Can you work these out from the model? Positions are in its coordinate system, mm. Give positions to 0.01 mm unless a question says otherwise; leave off trailing zeros. Loops run counter-clockwise (first coordinate to the right, second up) from the corner with the lowest first, then second, coordinate; pieces in that order, holes last. Notation, with made-up numbers: (-36, 37.25) -> (-5, 37.25) arc R37 cw to (-5, 76.25) -> close; hole circle Ø5 at (32, -20). An arc over 180 degrees is marked (long way). One line per question, with ' | ' between items.
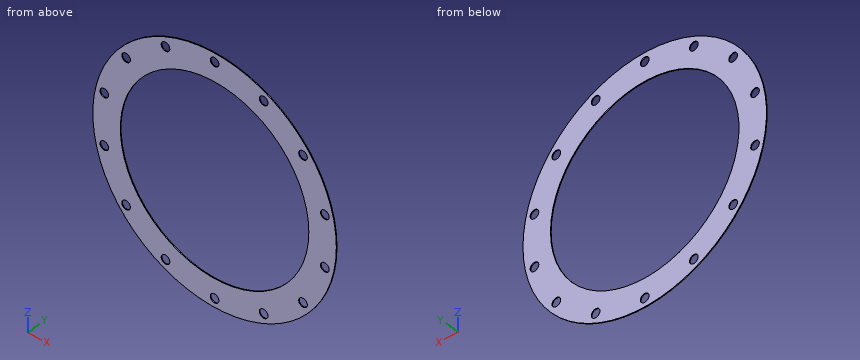
from build123d import *

# Parameters (mm, degrees)
F0_R     = 492.125
F0_R_2   = 17.4625
F0_R_3   = 381
F1_DEPTH = 3.175


with BuildPart() as f1:
    # F0 (on Front) → F1 (new body)
    with BuildSketch(Plane.XZ):
        Circle(F0_R)
        with Locations((-357.453354, -285.059537)):
            Circle(F0_R_2, mode=Mode.SUBTRACT)
        with Locations((-198.371646, -411.922966)):
            Circle(F0_R_2, mode=Mode.SUBTRACT)
        with Locations((0, -457.2)):
            Circle(F0_R_2, mode=Mode.SUBTRACT)
        with Locations((-445.737041, -101.736571)):
            Circle(F0_R_2, mode=Mode.SUBTRACT)
        Circle(F0_R_3, mode=Mode.SUBTRACT)
        with Locations((198.371646, -411.922966)):
            Circle(F0_R_2, mode=Mode.SUBTRACT)
        with Locations((357.453354, -285.059537)):
            Circle(F0_R_2, mode=Mode.SUBTRACT)
        with Locations((445.737041, -101.736571)):
            Circle(F0_R_2, mode=Mode.SUBTRACT)
        with Locations((-445.737041, 101.736571)):
            Circle(F0_R_2, mode=Mode.SUBTRACT)
        with Locations((-357.453354, 285.059537)):
            Circle(F0_R_2, mode=Mode.SUBTRACT)
        with Locations((-198.371646, 411.922966)):
            Circle(F0_R_2, mode=Mode.SUBTRACT)
        with Locations((0, 457.2)):
            Circle(F0_R_2, mode=Mode.SUBTRACT)
        with Locations((445.737041, 101.736571)):
            Circle(F0_R_2, mode=Mode.SUBTRACT)
        with Locations((198.371646, 411.922966)):
            Circle(F0_R_2, mode=Mode.SUBTRACT)
        with Locations((357.453354, 285.059537)):
            Circle(F0_R_2, mode=Mode.SUBTRACT)
    extrude(amount=F1_DEPTH)


solid = f1.part
Q1. If I drill on probe 1 along Z at (x, y) = (0, -2.5) (1 decimal); probe 2 along X at (y, z) = (-2.7, -425); probe 3 along X at (y, z) = (-1.4, 423), over which ranges is the centre line in solid material (lowest first)? Write a range as from..to.
Entries:
probe 1: -492.1..-474.7, -439.7..-381, 381..439.7, 474.7..492.1 | probe 2: -248.12..-209.94, -186.8..186.8, 209.94..248.12 | probe 3: -251.51..-211.87, -184.87..184.87, 211.87..251.51
Q2. If we section it at A-A (z = 0): Write out the boundary of the cut face in (x, y) (3 decimals), plus the area to 3 significant figures.
Entries:
outline: (-492.125, -3.175) -> (-381, -3.175) -> (-381, 0) -> (-492.125, 0) -> close; (381, -3.175) -> (492.125, -3.175) -> (492.125, 0) -> (381, 0) -> close | area: 706 mm²
Q3. If we section it at D-D (x = 297): Write out the boundary of the cut face in (y, z) (3 decimals), plus the area to 3 significant figures.
Entries:
outline: (-3.175, -392.4) -> (0, -392.4) -> (0, -238.646) -> (-3.175, -238.646) -> close; (-3.175, 238.646) -> (0, 238.646) -> (0, 392.4) -> (-3.175, 392.4) -> close | area: 976 mm²
Q4. If we section it at B-B (x = 0): Write out the boundary of the cut face in (y, z) (1 decimal), plus the area to 3 significant figures.
Entries:
outline: (-3.2, -492.1) -> (0, -492.1) -> (0, -474.7) -> (-3.2, -474.7) -> close; (-3.2, -439.7) -> (0, -439.7) -> (0, -381) -> (-3.2, -381) -> close; (-3.2, 381) -> (0, 381) -> (0, 439.7) -> (-3.2, 439.7) -> close; (-3.2, 474.7) -> (0, 474.7) -> (0, 492.1) -> (-3.2, 492.1) -> close | area: 484 mm²
Q5. If we section it at C-C (y = -1): State how many separate pieces and enclosed holes the cut face has, plus the area to 3 significant figures.
Entries:
separate pieces: 1 | enclosed holes: 15 | area: 291,000 mm²
Q6. For pin 1 Ø1 at (x, y) = (-156.5, -1) entering from -Z; pin 2 Ø21 at (x, z) = (357.45, -285.06) entering from +Y, each with a flat end and sliding along its axis, tell me the tip position at first contact or that it passes through.
Entries:
pin 1: z = -466.75 | pin 2: through
